Work out the finished part from the listing and answer in its coordinate system (mm). A direction names the side the tool comes from. Coordinates: 2 decimals unless noted, no trailing zeros. Order: outer loops, then holes, each group sorted by start corner. A loop starts at its lowest first (then second) coordinate and runs counter-clockwise, first axis right, second up.
1. The part is cut by section B-B, the plane y = 46. Give the vertices of the cut face in (x, z).
2. The part is cut by section A-A, the plane x = 102.5. Give the vertices of the cut face in (y, z).
3. The part is cut by section C-C, the plane z = 0. Give the vertices of the cut face in (x, y).
4. Flat-ended cylindrical pins translate along their axes: pin 1 Ø6 at (x, z) = (77, -9.5) entering from +Y; pin 2 Ø5 at (x, z) = (129.5, 1) entering from -Y; pin 3 Ø8 at (x, z) = (36, 5) entering from -Y. Find the tip coordinate at first contact, or state that the pin passes through.
5. Determine the mould class of faces 4 (the flat face through (73, 0, 24)), 5 (the flat face through (71, 16, -20)), 6 (the flat face through (144, 21, 0)) for opening direction X: +X half, -X half, draft (parallel to the pull), parting line (faces both ways), or undercut.
6. The part is cut by section D-D, the plane x = 23.5. Give the vertices of the cut face in (y, z).
7. A tool of negligible diameter and unlimited length cuts with its end or side. For faces 1 (the cylindrical face through (133.15, 16.48, 27.26)), 2 (the flat face through (133.15, 30.07, -20.42)), 3 (the cylindrical face through (110.93, 4.93, 22.65)), from which of +Z, -Z, +X, -X, +Y, -Y can it reach the whole face along a straight path? Write none if from no direction.
8. Find the intervals of material crossed by probe 1 along Z at (x, y) = (38, 3.25); probe 2 along X at (y, z) = (3.25, -22); probe 3 along Z at (x, y) = (108, 8), in increasing order.
```python
from build123d import *

# Parameters (mm, degrees)
BOSS_EXTRUDE1_DEPTH  = 32
SKETCH3_R            = 8
BOSS_EXTRUDE2_DEPTH  = 22
CUT_EXTRUDE1_DEPTH   = 145
LPATTERN1_COUNT      = 2
LPATTERN1_PITCH      = 70
LPATTERN1_COUNT_DIR2 = 2
LPATTERN1_PITCH_DIR2 = 44


with BuildPart() as part:
    # Sketch1 → Boss-Extrude1 (new body, symmetric)
    with BuildSketch(Plane.XY):
        Polygon((0, 0), (0, 36), (16, 52), (26, 52), (26, 16), (144, 16), (144, 0), align=None)
    extrude(amount=BOSS_EXTRUDE1_DEPTH, both=True)

    # Sketch3 → Boss-Extrude2 (add)
    with BuildSketch(Plane(origin=(144, 0, 0), x_dir=(0, 0, -1), z_dir=(1, 0, 0))):
        with BuildLine():
            Line((-14.500924593, 42.761892188), (-26.172487288, 17.732145215))
            ThreePointArc((-26.172487288, 17.732145215), (-27.279511824, 16.469825663), (-28.891410649, 16))
            Line((-28.891410649, 16), (28.891410649, 16))
            ThreePointArc((28.891410649, 16), (27.279511824, 16.469825663), (26.172487288, 17.732145215))
            Line((26.172487288, 17.732145215), (14.500924593, 42.761892188))
            ThreePointArc((14.500924593, 42.761892188), (0, 52), (-14.500924593, 42.761892188))
        make_face()
        with Locations((0, 36)):
            Circle(SKETCH3_R, mode=Mode.SUBTRACT)
    extrude(amount=-BOSS_EXTRUDE2_DEPTH)

    # Sketch4 → Cut-Extrude1 (cut, through all)
    with BuildSketch(Plane(origin=(144, 0, 0), x_dir=(0, 0, -1), z_dir=(1, 0, 0))):
        Polygon((-16, 0), (16, 0), (16, 7), (8, 7), (8, 16), (-8, 16), (-8, 7), (-16, 7), align=None)
    extrude(amount=-CUT_EXTRUDE1_DEPTH, mode=Mode.SUBTRACT)

    # Sketch6 → Ø6.0mm Dowel Hole1 (revolve, cut)
    with BuildSketch(Plane(origin=(38, 0, 22), x_dir=(0, 0, -1), z_dir=(1, 0, 0))):
        Polygon((0, 0), (0, 11.802581857), (3, 10), (3, 0), align=None)
    f_6_0mm_dowel_hole1 = revolve(axis=Axis((38, -6.35, 22), (0, 1, 0)), mode=Mode.SUBTRACT)

    # LPattern1: 6.0mm Dowel Hole1 2 × 2
    with Locations(*[(i * LPATTERN1_PITCH, 0, -j * LPATTERN1_PITCH_DIR2) for i in range(LPATTERN1_COUNT) for j in range(LPATTERN1_COUNT_DIR2) if (i, j) != (0, 0)]):
        add(f_6_0mm_dowel_hole1, mode=Mode.SUBTRACT)


solid = part.part
```
Geometry says:
1. outline: (10, -32) - (26, -32) - (26, 32) - (10, 32) - close; (122, -12.49) - (144, -12.49) - (144, 12.49) - (122, 12.49) - close
2. outline: (0, -32) - (16, -32) - (16, -8) - (7, -8) - (7, -16) - (0, -16) - close; (0, 16) - (7, 16) - (7, 8) - (16, 8) - (16, 32) - (0, 32) - close
3. outline: (0, 16) - (26, 16) - (26, 52) - (16, 52) - (0, 36) - close; (122, 16) - (144, 16) - (144, 28) - (122, 28) - close; (122, 44) - (144, 44) - (144, 52) - (122, 52) - close
4. pin 1: stops at y = 16
4. pin 2: stops at y = 16
4. pin 3: stops at y = 7
5. face 4: draft
5. face 5: undercut
5. face 6: +X half
6. outline: (0, -32) - (52, -32) - (52, 32) - (0, 32) - (0, 16) - (7, 16) - (7, 8) - (16, 8) - (16, -8) - (7, -8) - (7, -16) - (0, -16) - close
7. face 1: +Z, +X, +Y
7. face 2: -Z, +X, +Y
7. face 3: -Y
8. probe 1: z = -32 to -25, -19 to -16, 16 to 19, 25 to 32
8. probe 2: x = 0 to 35, 41 to 105, 111 to 144
8. probe 3: z = -32 to -25, -19 to -8, 8 to 19, 25 to 32
